Can you work these out from the model? Positions are in its coordinate system, mm. Face numbers are marked on the shaded views. A direction names the side the tool comes from. Give positions to 0.01 mm unless a question says otherwise; leave off trailing zeros. Loops run counter-clockwise (first coordinate to the right, second up) from the corner with the lowest first, then second, coordinate; pieces in that order, holes last. Notation, with made-up numbers: M 83.5,-4.75 L 125.5,-4.75 A30 cw 125.5,19.25 Z; hole C 10,54 d1. An arc over 180 degrees is marked long. Answer as a JSON object with one key per item and string values.
```python
from build123d import *

# Parameters (mm, degrees)
F0_R     = 23.426131
F1_DEPTH = 12.7
F2_R     = 16.876877
F3_DEPTH = 12.7
F4_R     = 11.09388
F5_DEPTH = 12.7


with BuildPart() as f1:
    # F0 (on Front) → F1 (new body)
    with BuildSketch(Plane.XZ):
        with Locations((0, 6.860897)):
            Circle(F0_R)
    extrude(amount=F1_DEPTH)

    # F2 (on face) → F3 (join)
    with BuildSketch(Plane.XZ.offset(12.7)):
        with Locations((0, 6.860897)):
            Circle(F2_R)
    extrude(amount=F3_DEPTH)

    # F4 (on face) → F5 (join)
    with BuildSketch(Plane.XZ.offset(25.4)):
        with Locations((0, 6.860897)):
            Circle(F4_R)
    extrude(amount=F5_DEPTH)


solid = f1.part
```
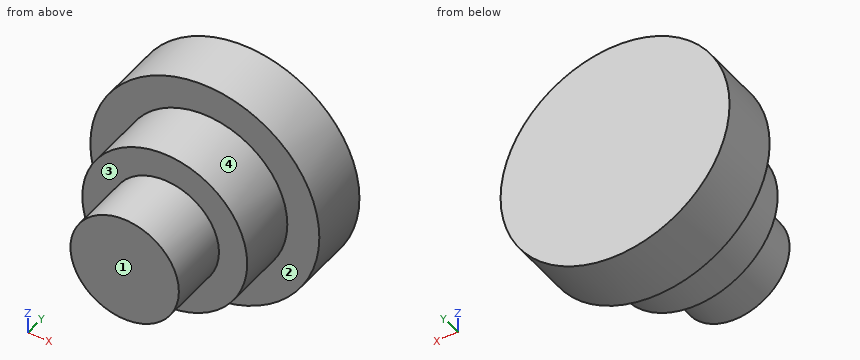
1) If we mould it in two halves opening along X, with no side actions, what happens to the marked faces 3 and 4? For each: +X half, -X half, draft (parallel to the pull), parting line (faces both ways), or undercut.
Answer list:
{"face 3": "draft", "face 4": "parting line"}
2) Suppose I cut it at B-B, the plane z = 2.5. Write out the boundary of the cut face in (x, y).
Answer list:
{"outline": "M -23.02,-12.7 L -16.3,-12.7 L -16.3,-25.4 L -10.2,-25.4 L -10.2,-38.1 L 10.2,-38.1 L 10.2,-25.4 L 16.3,-25.4 L 16.3,-12.7 L 23.02,-12.7 L 23.02,0 L -23.02,0 Z"}
3) Please list where these lines run through material, in increasing order: line 1 along Y through (x, z) = (-11.5, 6); line 2 along X through (y, z) = (-11, 27.5); line 3 along Y through (x, z) = (-18, 18.5). Write a range as from..to.
Answer list:
{"line 1": "-25.4..0", "line 2": "-11.08..11.08", "line 3": "-12.7..0"}
4) For the marked faces 1 and 2, which set-ups out of +Z, -Z, +X, -X, +Y, -Y let a thin tool reach every point of the face, with its end or its side?
Answer list:
{"face 1": "+Z, -Z, +X, -X, -Y", "face 2": "-Y"}
5) Suppose I cut it at D-D, the plane y = -23. Write out the boundary of the cut face in (x, z), and give its area (3 significant figures).
Answer list:
{"outline": "C 0,6.86 d33.75", "area": "895 mm^2"}
6) Will these pins go through, and if not, where does the flat tip stop? pin 1 Ø6 at (x, y) = (15, -22.5) entering from -Z; pin 2 Ø6 at (x, y) = (-7.5, -6) entering from -Z; pin 3 Ø1.5 at (x, y) = (-7.5, -29.5) entering from +Z.
Answer list:
{"pin 1": "z = -5.01", "pin 2": "z = -16.13", "pin 3": "z = 15.66"}
7) Suppose I cut it at C-C, the plane x = -15.5. Write out the boundary of the cut face in (y, z).
Answer list:
{"outline": "M -25.4,0.18 L -12.7,0.18 L -12.7,-10.7 L 0,-10.7 L 0,24.43 L -12.7,24.43 L -12.7,13.54 L -25.4,13.54 Z"}
8) Suppose I cut it at A-A, the plane x = 0. Write out the boundary of the cut face in (y, z), and give its area (3 significant figures).
Answer list:
{"outline": "M -38.1,-4.23 L -25.4,-4.23 L -25.4,-10.02 L -12.7,-10.02 L -12.7,-16.57 L 0,-16.57 L 0,30.29 L -12.7,30.29 L -12.7,23.74 L -25.4,23.74 L -25.4,17.95 L -38.1,17.95 Z", "area": "1,310 mm^2"}
